Here's the drawing with two shaded views (mm, measured from the low corner). I have some questions. Round coordinates to 2 decimals unless told otherwise and drop trailing zeros. Order: outer loops, then holes, each group sorted by start corner. A loop starts at its lowest first (then second) coordinate and runs counter-clockwise, first axis right, second up.
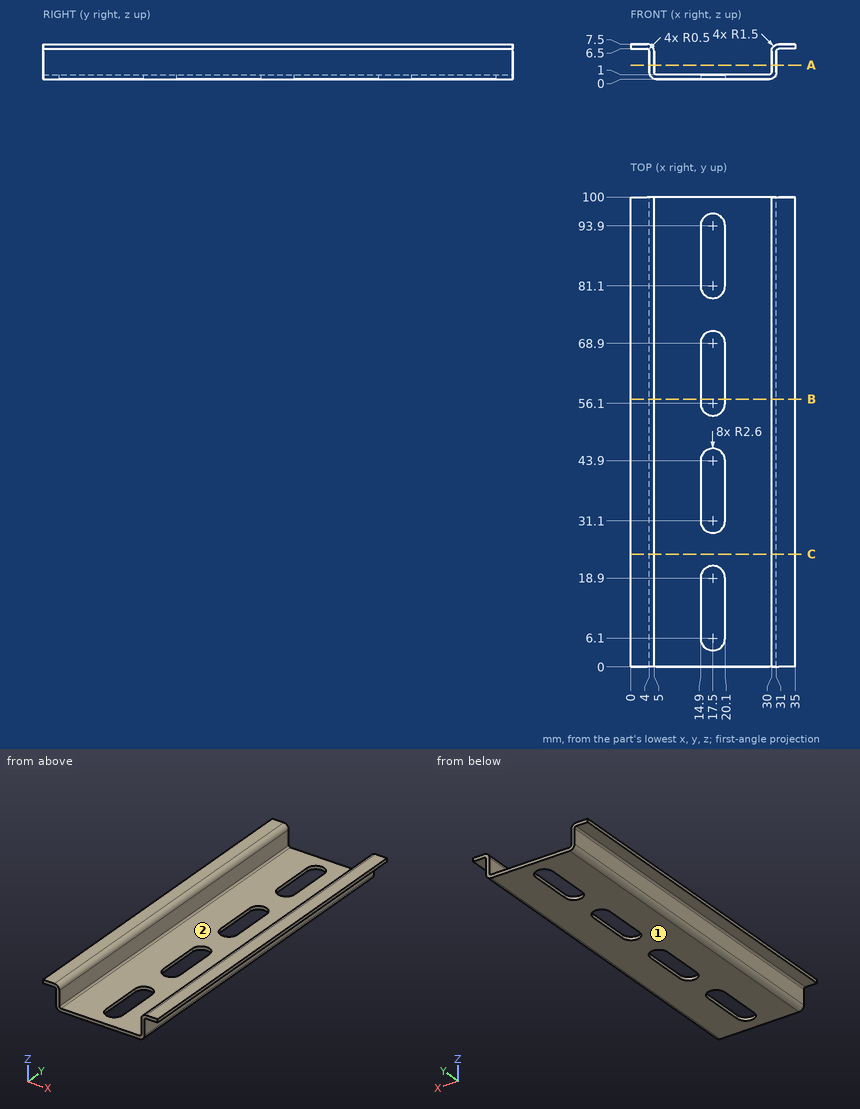
1. I'm going to push flat-ended pins straight in: P1, Ø3.5, axis at y = 56, z = 4.5, coming from the +X side; P2, Ø1.1, axis at y = 40, z = 0.5, coming from the -X side; P3, Ø3.5, axis at y = 37.5, z = 4, coming from the -X side. Where does each tip first touch, or does it pass through?
Evaluation:
P1: stops at x = 31.07
P2: stops at x = 4.07
P3: stops at x = 4
2. I need wall thicknesses on probe 1 along X at (y, z) = (21.5, 3); probe 2 along Z at (x, y) = (11, 4); probe 3 along Z at (x, y) = (32, 62.5). Which ranges of each line are inside material? Lowest first, please.
Evaluation:
probe 1: x = 4 to 5, 30 to 31
probe 2: z = 0 to 1
probe 3: z = 6.5 to 7.5
3. If we mould it in two halves opening along X, with no side actions, what happens to the marked faces 1 and 2? For each: released by +X, released by -X, zero draft, split by the parting line, or undercut.
Evaluation:
face 1: zero draft
face 2: undercut
4. If we section it at B-B, the plane y = 57: Write out the boundary of the cut face in (x, z).
Evaluation:
outline: (0, 6.5) - (3.5, 6.5) arc R0.5 cw to (4, 6) - (4, 1.5) arc R1.5 ccw to (5.5, 0) - (14.9, 0) - (14.9, 1) - (5.5, 1) arc R0.5 cw to (5, 1.5) - (5, 6) arc R1.5 ccw to (3.5, 7.5) - (0, 7.5) - close; (20.1, 0) - (29.5, 0) arc R1.5 ccw to (31, 1.5) - (31, 6) arc R0.5 cw to (31.5, 6.5) - (35, 6.5) - (35, 7.5) - (31.5, 7.5) arc R1.5 ccw to (30, 6) - (30, 1.5) arc R0.5 cw to (29.5, 1) - (20.1, 1) - close
5. If we section it at A-A, the plane z = 3: Write out the boundary of the cut face in (x, y), and give its area (3 significant figures).
Evaluation:
outline: (4, 0) - (5, 0) - (5, 100) - (4, 100) - close; (30, 0) - (31, 0) - (31, 100) - (30, 100) - close
area: 200 mm2
6. If we section it at C-C, the plane y = 24: Write out the boundary of the cut face in (x, z), and give its area (3 significant figures).
Evaluation:
outline: (0, 6.5) - (3.5, 6.5) arc R0.5 cw to (4, 6) - (4, 1.5) arc R1.5 ccw to (5.5, 0) - (29.5, 0) arc R1.5 ccw to (31, 1.5) - (31, 6) arc R0.5 cw to (31.5, 6.5) - (35, 6.5) - (35, 7.5) - (31.5, 7.5) arc R1.5 ccw to (30, 6) - (30, 1.5) arc R0.5 cw to (29.5, 1) - (5.5, 1) arc R0.5 cw to (5, 1.5) - (5, 6) arc R1.5 ccw to (3.5, 7.5) - (0, 7.5) - close
area: 46.3 mm2
